```python
from build123d import *

# Parameters (mm, degrees)
SM_BASE_FLANGE_2_DEPTH = 25
M6X1_01_D              = 5
M6X1_01_CSINK_D        = 6.5
M6X1_01_CSINK_ANGLE    = 90
CHAMFER_1_SIZE         = 7


# Sheet-metal steps are written as plain solids
with BuildPart() as part:
    # Sketch 2 → Базовая кромка2 (new, symmetric)
    with BuildSketch(Plane(origin=(0, 0, 0), x_dir=(1, 0, 0), z_dir=(0, 1, 0))):
        with BuildLine():
            Line((-365.5, 87), (-365.5, 61.551362713))
            ThreePointArc((-365.5, 61.551362713), (-363.846826722, 56.681271281), (-359.570552361, 53.823956103))
            Line((-359.570552361, 53.823956103), (-189.570552361, 8.27259339))
            ThreePointArc((-189.570552361, 8.27259339), (-188.544209538, 8.068441109), (-187.5, 8))
            Line((-187.5, 8), (187.5, 8))
            ThreePointArc((187.5, 8), (188.544209538, 8.068441109), (189.570552361, 8.27259339))
            Line((189.570552361, 8.27259339), (359.570552361, 53.823956103))
            ThreePointArc((359.570552361, 53.823956103), (363.846826722, 56.681271281), (365.5, 61.551362713))
            Line((365.5, 61.551362713), (365.5, 87))
            Line((365.5, 87), (373.5, 87))
            Line((373.5, 87), (373.5, 61.551362713))
            ThreePointArc((373.5, 61.551362713), (370.193653445, 51.811179849), (361.641104722, 46.096549493))
            Line((361.641104722, 46.096549493), (191.641104722, 0.545186779))
            ThreePointArc((191.641104722, 0.545186779), (189.588419076, 0.136882218), (187.5, 0))
            Line((187.5, 0), (-187.5, 0))
            ThreePointArc((-187.5, 0), (-189.588419076, 0.136882218), (-191.641104722, 0.545186779))
            Line((-191.641104722, 0.545186779), (-361.641104722, 46.096549493))
            ThreePointArc((-361.641104722, 46.096549493), (-370.193653445, 51.811179849), (-373.5, 61.551362713))
            Line((-373.5, 61.551362713), (-373.5, 87))
            Line((-373.5, 87), (-365.5, 87))
        make_face()
    extrude(amount=SM_BASE_FLANGE_2_DEPTH, both=True)

    # Отверстие обработанное метчиком M6x1.01 (through all)
    with Locations(Plane(origin=(175, 12.5, -8), x_dir=(-1, 0, 0), z_dir=(0, 0, -1))):
        with Locations((0, 0), (25, 0), (25, -25), (0, -25), (325, 0), (350, 0), (350, -25), (325, -25)):
            CounterSinkHole(M6X1_01_D / 2, M6X1_01_CSINK_D / 2, counter_sink_angle=M6X1_01_CSINK_ANGLE)

    # Фаска1
    chamfer_1_edges = [part.edges().sort_by_distance(p)[0] for p in [
        (369.5, -25, -87),
        (-369.5, -25, -87),
    ]]
    chamfer(chamfer_1_edges, length=CHAMFER_1_SIZE)


solid = part.part
```
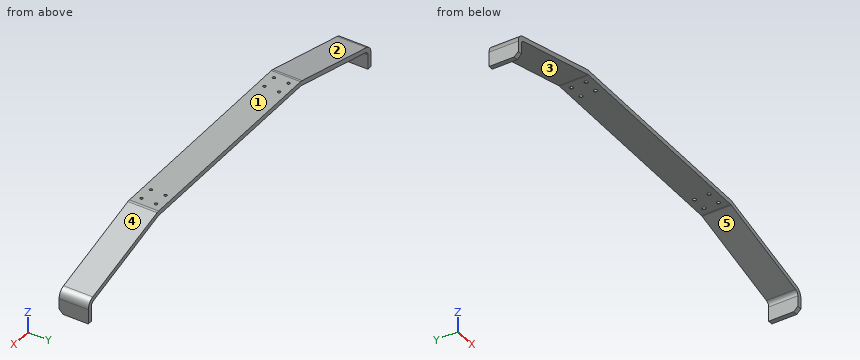
Can you work these out from the model? Positions are in its coordinate system, mm. Face numbers are marked on the shaded views. A direction names the side the tool comes from. Coordinates: 2 decimals unless noted, no trailing zeros. Write each loop counter-clockwise with the first axis right and the second up, starting at its lowest first coordinate (ties: lowest second). Pieces come first, ordered by that corner, then holes. Notation, with made-up numbers: M -37,-36 L 3,-36 A10 cw 3,-27 Z; hole C -35,80.25 d3. An arc over 180 degrees is marked long. Answer as CSV lines item,"result".
Item 1: Imagine slicing it at B-B on x = 93. List the corners of the cut face in (y, z) for me, plus the area to 3 significant figures.
Geometry results:
outline,"M -25,-8 L 25,-8 L 25,0 L -25,0 Z"
area,"400 mm2"
Item 2: Imagine slicing it at C-C on x = -268. List the corners of the cut face in (y, z) for me, plus the area to 3 significant figures.
Geometry results:
outline,"M -25,-29.29 L 25,-29.29 L 25,-21.01 L -25,-21.01 Z"
area,"414 mm2"
Item 3: I'm going to push flat-ended pins straight in: P1, Ø4, axis at x = 150, y = -12.5, coming from the -Z side; P2, Ø8, axis at x = -280.5, y = -4.5, coming from the +Z side; P3, Ø6, axis at x = 150, y = 12.5, coming from the -Z side; P4, Ø8, axis at x = -175, y = 12.5, coming from the -Z side. Where does each tip first touch, or does it pass through?
Geometry results:
P1,"passes through"
P2,"stops at z = -23.28"
P3,"stops at z = -7.75"
P4,"stops at z = -8"
Item 4: We'd pull the mould along X, two halves only. Please class the marked faces 1, 2 and 3: +X half, -X half, draft (parallel to the pull), parting line (faces both ways), or undercut.
Geometry results:
face 1,"draft"
face 2,"-X half"
face 3,"undercut"
Item 5: On a 3-axis mill with a long thin cutter (end or side, diameter ignored), from which of +Z, -Z, +X, -X, +Y, -Y can I reach the whole of each face in a straight line? I mean the marked faces 4 and 5. Say none if no direction works.
Geometry results:
face 4,"+Z, +X, +Y, -Y"
face 5,"-Z, +Y, -Y"
Item 6: Please list where these lines run through material, in increasing order: line 1 along Y through (x, z) = (150, -4); line 2 along Z through (x, y) = (30, 20.5); line 3 along Z through (x, y) = (-335, 2).
Geometry results:
line 1,"y = -25 to -15, -10 to 10, 15 to 25"
line 2,"z = -8 to 0"
line 3,"z = -47.24 to -38.96"
Item 7: Imagine slicing it at A-A on z = -24.5. List the corners of the cut face in (x, y) for me.
Geometry results:
outline,"M -281.04,-25 L -250.13,-25 L -250.13,25 L -281.04,25 Z; M 250.13,-25 L 281.04,-25 L 281.04,25 L 250.13,25 Z"
